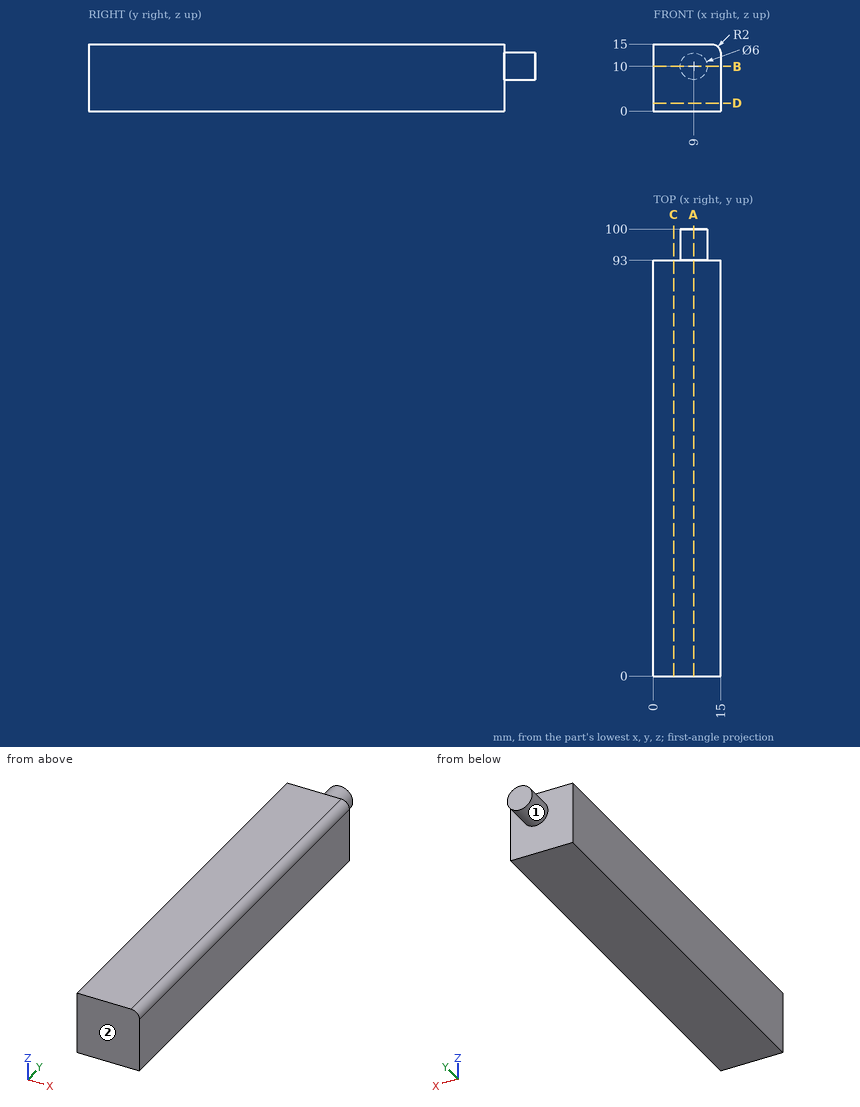
Here's the drawing with two shaded views (mm, measured from the low corner). I have some questions. A direction names the side the tool comes from. Round coordinates to 2 decimals unless told otherwise and drop trailing zeros. Order: outer loops, then holes, each group sorted by start corner. A loop starts at its lowest first (then second) coordinate and runs counter-clockwise, first axis right, second up. Notation, with made-up numbers: (-29, -17) -> (-13, -17) arc R28 ccw to (-13, 14) -> close; hole circle Ø7 at (-11.5, 83). An arc over 180 degrees is marked (long way). Return JSON: item names as keys, results as strings.
Q1. If we section it at A-A on x = 9: List the corners of the cut face in (y, z) for me.
Filled sheet:
{"outline": "(0, 0) -> (93, 0) -> (93, 7) -> (100, 7) -> (100, 13) -> (93, 13) -> (93, 15) -> (0, 15) -> close"}
Q2. I need wall thicknesses on line 1 along Y through (x, z) = (8, 1.5); line 2 along X through (y, z) = (13, 13.25). Which ranges of each line are inside material? Lowest first, please. Write a range as from..to.
Filled sheet:
{"line 1": "y = 0..93", "line 2": "x = 0..14.98"}
Q3. For pin 1 Ø4.5 at (x, z) = (5, 4.5) entering from +Y, with a flat end and sliding along its axis, tell me the tip position at first contact or that it passes through.
Filled sheet:
{"pin 1": "stops at y = 93"}
Q4. Which directions (+Z, -Z, +X, -X, +Y, -Y) give clear straight access to the entire face, cutting with the end or side of a thin tool? Please do the marked faces 1 and 2.
Filled sheet:
{"face 1": "+Y", "face 2": "+Z, -Z, +X, -X, -Y"}
Q5. If we section it at D-D on z = 1.75: List the corners of the cut face in (x, y) for me, plus the area to 4 significant figures.
Filled sheet:
{"outline": "(0, 0) -> (15, 0) -> (15, 93) -> (0, 93) -> close", "area": "1,395 mm^2"}
Q6. If we section it at C-C on x = 4.5: List the corners of the cut face in (y, z) for me.
Filled sheet:
{"outline": "(0, 0) -> (93, 0) -> (93, 15) -> (0, 15) -> close"}
Q7. If we section it at B-B on z = 10: List the corners of the cut face in (x, y) for me, plus the area to 3 significant figures.
Filled sheet:
{"outline": "(0, 0) -> (15, 0) -> (15, 93) -> (12, 93) -> (12, 100) -> (6, 100) -> (6, 93) -> (0, 93) -> close", "area": "1,440 mm^2"}
